Geometry: final body of the model. Coordinates: model frame, mm. Give positions to 0.01 mm unless a question says otherwise; leave off trailing zeros. Write each loop counter-clockwise with the first axis right and the second up, starting at its lowest first coordinate (ties: lowest second). Pieces come first, ordered by that corner, then holes. Notation, with made-up numbers: M 7,76.5 L 54,76.5 A13 cw 54,95.5 Z; hole C -20,-20.75 d4. An arc over 180 degrees is marked long. Use a Markdown table: item, result. Add a question column.
(1) Cut plane B-B (z = -5.08). Output: boundary loops of the cut face in (x, y).
(2) Cut plane D-D (x = 3.5). Output: boundary loops of the cut face in (y, z).
(3) Material intervals for L1, parallel to Z at x = 1, y = -0.4; L2, parallel to Z at x = 3.5, y = -0.2, sorted ascending.
(4) Cut plane A-A (x = 1.27). Output: boundary loops of the cut face in (y, z).
(5) Draft query along Z for faces 1 (the cylindrical face through (-5.978, 0.011, 4.675)), 2 (the flat face through (0, 0.8, 0)), 3 (the flat face through (0, 0, 6.35)). Return one class per face: released by +Z, released by -Z, zero draft, split by the parting line, or undercut.
(6) Cut plane C-C (y = 0.45). State how many separate pieces and enclosed holes the cut face has, plus the area to 3 significant figures.
(7) Pin query (flat end, axial travel): pin 1 Ø0.7 at (x, z) = (-6.35, -5.08) entering from -Y (3 decimals). Return the tip coordinate at first contact, or that it passes through.
```python
from build123d import *

# Parameters (mm, degrees)
SKETCH1_W            = 15.24
SKETCH1_H            = 12.7
BOSS_EXTRUDE1_DEPTH  = 0.8
SKETCH2_R            = 0.55
CUT_EXTRUDE1_DEPTH   = 11.04723345
LPATTERN1_COUNT      = 6
LPATTERN1_PITCH      = 2.54
LPATTERN1_COUNT_DIR2 = 2
LPATTERN1_PITCH_DIR2 = 10.16


with BuildPart() as part:
    # Sketch1 → Boss-Extrude1 (new, symmetric)
    with BuildSketch(Plane(origin=(0, 0, 0), x_dir=(1, 0, 0), z_dir=(0, 1, 0))):
        Rectangle(SKETCH1_W, SKETCH1_H)
    extrude(amount=BOSS_EXTRUDE1_DEPTH, both=True)

    # Sketch2 → Cut-Extrude1 (cut, through all)
    with BuildSketch(Plane(origin=(0, 0.8, 0), x_dir=(1, 0, 0), z_dir=(0, 1, 0))):
        with Locations(Location((-6.35, -5.08, 0), (0, 0, 270))):
            Circle(SKETCH2_R)
    cut_extrude1 = extrude(amount=-CUT_EXTRUDE1_DEPTH, mode=Mode.SUBTRACT)

    # LPattern1: Cut-Extrude1 6 × 2
    with Locations(*[(i * LPATTERN1_PITCH, 0, -j * LPATTERN1_PITCH_DIR2) for i in range(LPATTERN1_COUNT) for j in range(LPATTERN1_COUNT_DIR2) if (i, j) != (0, 0)]):
        add(cut_extrude1, mode=Mode.SUBTRACT)


solid = part.part
```
Answer list:
| question | item | result |
|---|---|---|
| 1 | outline | M -7.62,-0.8 L -6.9,-0.8 L -6.9,0.8 L -7.62,0.8 Z; M -5.8,-0.8 L -4.36,-0.8 L -4.36,0.8 L -5.8,0.8 Z; M -3.26,-0.8 L -1.82,-0.8 L -1.82,0.8 L -3.26,0.8 Z; M -0.72,-0.8 L 0.72,-0.8 L 0.72,0.8 L -0.72,0.8 Z; M 1.82,-0.8 L 3.26,-0.8 L 3.26,0.8 L 1.82,0.8 Z; M 4.36,-0.8 L 5.8,-0.8 L 5.8,0.8 L 4.36,0.8 Z; M 6.9,-0.8 L 7.62,-0.8 L 7.62,0.8 L 6.9,0.8 Z |
| 2 | outline | M -0.8,-6.35 L 0.8,-6.35 L 0.8,-5.53 L -0.8,-5.53 Z; M -0.8,-4.63 L 0.8,-4.63 L 0.8,4.63 L -0.8,4.63 Z; M -0.8,5.53 L 0.8,5.53 L 0.8,6.35 L -0.8,6.35 Z |
| 3 | L1 | -6.35 to -5.56, -4.6 to 4.6, 5.56 to 6.35 |
| 3 | L2 | -6.35 to -5.53, -4.63 to 4.63, 5.53 to 6.35 |
| 4 | outline | M -0.8,-6.35 L 0.8,-6.35 L 0.8,-5.63 L -0.8,-5.63 Z; M -0.8,-4.53 L 0.8,-4.53 L 0.8,4.53 L -0.8,4.53 Z; M -0.8,5.63 L 0.8,5.63 L 0.8,6.35 L -0.8,6.35 Z |
| 5 | face 1 | undercut |
| 5 | face 2 | zero draft |
| 5 | face 3 | released by +Z |
| 6 | separate pieces | 1 |
| 6 | enclosed holes | 12 |
| 6 | area | 182 mm² |
| 7 | pin 1 | through |
